```python
from build123d import *

# Parameters (mm, degrees)
FACE_2_DEPTH           = 5
SKETCH2_W              = 14.632926246
SKETCH2_H              = 5
BOSS_EXTRUDE2_DEPTH    = 7
SKETCH3_W              = 14.632926246
SKETCH3_H              = 7
BOSS_EXTRUDE3_DEPTH    = 7
EYE_HOLES_REACH        = 248.075
SKETCH4_R              = 1.15
SKETCH5_W              = 14.632926246
SKETCH5_H              = 3.5
SEAT_DEPTH             = 7
SKETCH6_W              = 18
SKETCH6_H              = 5
BOSS_EXTRUDE4_DEPTH    = 3.5
SKETCH7_W              = 18.025006546
SKETCH7_H              = 4.25
TOP_HOLE_DEPTH         = 248.972829901
MIDDLE_HOLE_DEPTH      = 246.672789516
MIDDLE_HOLE_DEPTH_BACK = 246.672789516
SKETCH8_R              = 5.003684601
SKETCH11_R             = 0.754398486
CUT_EXTRUDE9_DEPTH     = 246.672789516


with BuildPart() as part:
    # Sketch1 → Face 2 (new body)
    with BuildSketch(Plane.XY):
        Polygon((189.199131389, 129.336090234), (189.219408928, 129.168352428), (189.276625012, 129.01501095), (189.375109043, 128.870497126), (189.879763338, 128.333185306), (190.417075159, 127.828531011), (190.558185088, 127.731803407), (190.715733881, 127.672634267), (190.882668266, 127.652553357), (205.515594512, 127.652553357), (205.683332318, 127.672830896), (205.84007769, 127.731803407), (205.98118762, 127.828531011), (207.023153735, 128.870497126), (207.118523911, 129.009007135), (207.17885385, 129.168352428), (207.199131389, 129.336090234), (207.199131389, 132.202042434), (189.199131389, 132.202042434), align=None)
    extrude(amount=FACE_2_DEPTH)

    # Sketch2 → Boss-Extrude2 (add)
    with BuildSketch(Plane.XZ.offset(-127.652553357)):
        with Locations((198.199131389, 2.5)):
            Rectangle(SKETCH2_W, SKETCH2_H)
    extrude(amount=BOSS_EXTRUDE2_DEPTH)

    # Sketch3 → Boss-Extrude3 (add)
    with BuildSketch(Plane(origin=(0, 0, 0), x_dir=(-1, 0, 0), z_dir=(0, 0, -1))):
        with Locations((-198.199131389, 124.152553357)):
            Rectangle(SKETCH3_W, SKETCH3_H)
    extrude(amount=BOSS_EXTRUDE3_DEPTH)

    # Sketch4 → Eye Holes (cut, up to next)
    with BuildSketch(Plane.XY.offset(5), mode=Mode.PRIVATE) as eye_holes_sk1:
        with Locations((191.649131389, 129.852042434)):
            Circle(SKETCH4_R)
    eye_holes_tool1 = extrude(eye_holes_sk1.sketch, amount=-EYE_HOLES_REACH, mode=Mode.PRIVATE) & part.part
    # Sketch4 → Eye Holes (cut, up to next)
    with BuildSketch(Plane.XY.offset(5), mode=Mode.PRIVATE) as eye_holes_sk2:
        with Locations((204.599131389, 129.852042434)):
            Circle(SKETCH4_R)
    eye_holes_tool2 = extrude(eye_holes_sk2.sketch, amount=-EYE_HOLES_REACH, mode=Mode.PRIVATE) & part.part
    add(eye_holes_tool1.solids().sort_by_distance((191.649131, 129.852042, 5))[0], mode=Mode.SUBTRACT)
    add(eye_holes_tool2.solids().sort_by_distance((204.599131, 129.852042, 5))[0], mode=Mode.SUBTRACT)

    # Sketch5 → Seat (cut)
    with BuildSketch(Plane(origin=(0, 0, -7), x_dir=(-1, 0, 0), z_dir=(0, 0, -1))):
        with Locations((-198.199131389, 125.902553357)):
            Rectangle(SKETCH5_W, SKETCH5_H)
    extrude(amount=-SEAT_DEPTH, mode=Mode.SUBTRACT)

    # Sketch6 → Boss-Extrude4 (add)
    with BuildSketch(Plane(origin=(0, 132.202042434, 0), x_dir=(1, 0, 0), z_dir=(0, 1, 0))):
        with Locations((198.199131389, -2.5)):
            Rectangle(SKETCH6_W, SKETCH6_H)
    extrude(amount=BOSS_EXTRUDE4_DEPTH)

    # Sketch7 → Top Hole (cut, through all)
    with BuildSketch(Plane.XY.offset(5)):
        with Locations((198.194207579, 133.577042434)):
            Rectangle(SKETCH7_W, SKETCH7_H)
    extrude(amount=-TOP_HOLE_DEPTH, mode=Mode.SUBTRACT)

    # Sketch8 → Middle Hole (cut, two sides: drawn at the far end of the back side and taken through both)
    with BuildSketch(Plane.XY.offset(5).offset(-MIDDLE_HOLE_DEPTH_BACK)):
        with Locations((198.199131389, 131.452042434)):
            Circle(SKETCH8_R)
    extrude(amount=MIDDLE_HOLE_DEPTH + MIDDLE_HOLE_DEPTH_BACK, mode=Mode.SUBTRACT)

    # Sketch11 → Cut-Extrude9 (cut, through all)
    with BuildSketch(Plane.XY.offset(5)):
        with Locations((192.88691871, 131.452042434)):
            Circle(SKETCH11_R)
        with Locations((202.919958348, 131.377258625)):
            Circle(SKETCH11_R)
    extrude(amount=-CUT_EXTRUDE9_DEPTH, mode=Mode.SUBTRACT)


solid = part.part
```
Part model, mm, in its own coordinate system. A direction names the side the tool comes from. Round coordinates to 2 decimals unless told otherwise and drop trailing zeros. Order: outer loops, then holes, each group sorted by start corner. A loop starts at its lowest first (then second) coordinate and runs counter-clockwise, first axis right, second up. Notation, with made-up numbers: M 32,-7.75 L 71,-7.75 A23 cw 71,24.25 Z; hole C -33,1 d7. An arc over 180 degrees is marked long. Answer in a Markdown table with one row per item. Add a question column.
Q1. Cut at D-D on z = 1.5. Give the cut face in (x, y).
Q2. Cut at C-C on z = -5. Give the cut face in (x, y).
Q3. Cut at B-B on y = 126.75. Give the cut face in (x, z).
Q4. Wall check: L1, parallel to Y at x = 204.5, z = 4.5; L2, parallel to X at y = 125.75, z = 4; L3, parallel to X at y = 129.75, z = 3.75. Give the ranges that are in metal, low to high. Write a range as from..to.
Q5. 3-axis set-ups, long thin cutter, end or side, ignore diameter. For faces 4 (the face through (198, 122, -7)), 5 (the face through (205.516, 123, 0)), 6 (the face through (198, 124.153, -4)): which of +Z, -Z, +X, -X, +Y, -Y reach the whole face in a straight line?
Q6. Pin check, flat tips, straight feed: pin 1 (5 mm diameter, centred on y = 123, z = -1.5, fed in from -X); pin 2 (1.5 mm diameter, centred on y = 127.5, z = 2, fed in from +X); pin 3 (1.4 mm diameter, centred on x = 191.65, y = 129.85, fed in from -Z); pin 4 (2 mm diameter, centred on x = 201.5, z = -5, fed in from +Y). Stop position of each tip, or through.
Q7. Mould opens along X. For faces 1 (the face through (190.883, 123, 0)), 2 (the face through (198, 120.653, -1)), 3 (the face through (204.449, 130.992, 2.535)) say: +X half, -X half, draft (parallel to the pull), parting line (faces both ways), or undercut.
Q8. Cut at A-A on x = 205. Give the cut face in (y, z), and give its area (3 significant figures).
Established:
| question | item | result |
|---|---|---|
| 1 | outline | M 189.2,129.34 L 189.22,129.17 L 189.28,129.02 L 189.38,128.87 L 189.88,128.33 L 190.42,127.83 L 190.56,127.73 L 190.72,127.67 L 190.88,127.65 L 190.88,120.65 L 205.52,120.65 L 205.52,127.65 L 205.68,127.67 L 205.84,127.73 L 205.98,127.83 L 207.02,128.87 L 207.12,129.01 L 207.18,129.17 L 207.2,129.34 L 207.2,131.45 L 203.67,131.45 A0.75 cw 203.14,130.66 A5 cw 193.24,130.79 A0.75 cw 192.13,131.45 L 189.2,131.45 Z; hole C 191.65,129.85 d2.3; hole C 204.6,129.85 d2.3 |
| 2 | outline | M 190.88,120.65 L 205.52,120.65 L 205.52,124.15 L 190.88,124.15 Z |
| 3 | outline | M 190.88,0 L 196.49,0 L 196.49,5 L 190.88,5 Z; M 199.91,0 L 205.52,0 L 205.52,5 L 199.91,5 Z |
| 4 | L1 | y = 120.65..128.71, 131..131.45 |
| 4 | L2 | x = 190.88..205.52 |
| 4 | L3 | x = 189.2..190.5, 192.79..193.49, 202.9..203.45, 205.74..207.2 |
| 5 | face 4 | -Z, +X, -X, +Y, -Y |
| 5 | face 5 | +Z, -Z, +X, -Y |
| 5 | face 6 | -Z, +X, -X, +Y |
| 6 | pin 1 | stops at x = 190.88 |
| 6 | pin 2 | stops at x = 206.4 |
| 6 | pin 3 | passes through |
| 6 | pin 4 | stops at y = 124.15 |
| 7 | face 1 | -X half |
| 7 | face 2 | draft |
| 7 | face 3 | undercut |
| 8 | outline | M 120.65,-7 L 124.15,-7 L 124.15,0 L 128.77,0 L 128.77,5 L 120.65,5 Z; M 130.93,0 L 131.45,0 L 131.45,5 L 130.93,5 Z |
| 8 | area | 67.7 mm2 |
